Input: part model. Units: mm. Frame: model coordinates. Face numbers are marked on the shaded views. A direction names the side the tool comes from. Give positions to 0.01 mm unless a question says otherwise; leave off trailing zeros. Write each loop counter-clockwise with the first axis right and the second up, starting at its lowest first coordinate (ties: lowest second). Pieces come first, ordered by that corner, then holes. Notation, with made-up numbers: (53.5, 58) - (108.5, 58) arc R20 ccw to (108.5, 85) - close; hole circle Ø3 at (79, -39). An arc over 180 degrees is marked (long way). Use a Markdown table: item, result. Add a question column.
1. Material intervals for probe 1 along Y at (x, z) = (0, -8.75); probe 2 along X at (y, z) = (-0.75, -11.25); probe 3 along Y at (x, z) = (1, -0.5), sorted ascending.
2. Pin query (flat end, axial travel): pin 1 (1.2 mm diameter, centred on x = 0, z = -1, fed in from -Y); pin 2 (3 mm diameter, centred on x = 0, z = -7, fed in from +Y); pin 3 (0.9 mm diameter, centred on x = 0, z = -1, fed in from +Y). Return the tip coordinate at first contact, or that it passes through.
3. Section query B-B, the plane z = -7. Return loops of the section in (x, y), plus the area to 3 significant figures.
4. Mould query, pull axis Y, two halves, no side actions, for the marked faces 3, 4 and 5. Classes: released by +Y, released by -Y, zero draft, split by the parting line, or undercut.
5. Set-up query: the marked faces 1 and 2. Return all of +Z, -Z, +X, -X, +Y, -Y with unobstructed straight access to the full face (end or side cutting, diameter ignored); none if empty.
```python
from build123d import *

# Parameters (mm, degrees)
SKETCH001_R     = 2.15
POCKET_DEPTH    = 3.119566
CHAMFER_SIZE    = 0.25
CHAMFER001_SIZE = 0.2


with BuildPart() as pocket:
    # Sketch003 → Revolution001 (revolve)
    with BuildSketch(Plane.XZ):
        Polygon((0, -2.118566), (1.15, -1.7), (1.15, 1), (0, 1), align=None)
    revolve(axis=Axis((0, 0, 0), (0, 0, 1)))

    # Sketch001 → Pocket (cut, through all)
    with BuildSketch(Plane(origin=(0, 0, 1), x_dir=(-1, 0, 0), z_dir=(0, 0, 1))):
        Circle(SKETCH001_R)
        Polygon((-0.57735, 1), (0.57735, 1), (1.154701, 0), (0.57735, -1), (-0.57735, -1), (-1.154701, 0), align=None, mode=Mode.SUBTRACT)
    extrude(amount=-POCKET_DEPTH, mode=Mode.SUBTRACT)


with BuildPart() as chamfer001:
    # Sketch → Revolution (revolve)
    with BuildSketch(Plane.XZ):
        Polygon((1.15, 0), (3.199999, 0), (1.5, -1.7), (1.5, -12), (0, -12), (0, -1.150001), align=None)
    revolve(axis=Axis((0, 0, 0), (0, 0, 1)))

    # Cut: cut Pocket
    add(pocket.part, mode=Mode.SUBTRACT)

    # Chamfer
    chamfer_edges = [chamfer001.edges().sort_by_distance(p)[0] for p in [
        (-3.199999, 0, 0),
    ]]
    chamfer(chamfer_edges, length=CHAMFER_SIZE)

    # Chamfer001
    chamfer001_edges = [chamfer001.edges().sort_by_distance(p)[0] for p in [
        (-1.5, 0, -12),
    ]]
    chamfer(chamfer001_edges, length=CHAMFER001_SIZE)


solid = chamfer001.part
```
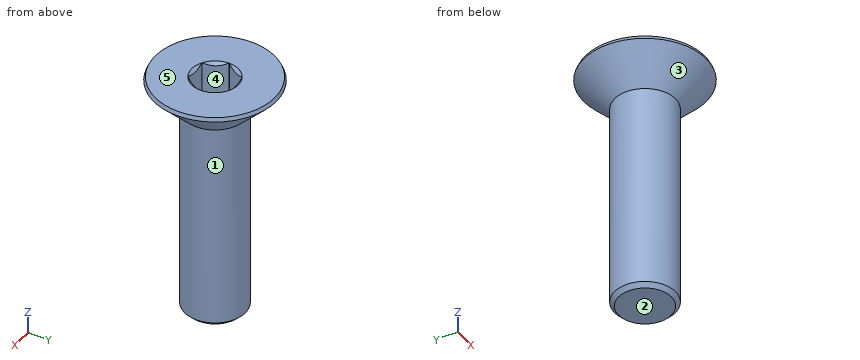
Result sheet:
| question | item | result |
|---|---|---|
| 1 | probe 1 | y = -1.5 to 1.5 |
| 1 | probe 2 | x = -1.3 to 1.3 |
| 1 | probe 3 | y = -2.51 to -0.27, 0.27 to 2.51 |
| 2 | pin 1 | stops at y = -2.8 |
| 2 | pin 2 | stops at y = 1.5 |
| 2 | pin 3 | stops at y = 2.65 |
| 3 | outline | circle Ø3 at (0, 0) |
| 3 | area | 7.07 mm² |
| 4 | face 3 | split by the parting line |
| 4 | face 4 | undercut |
| 4 | face 5 | zero draft |
| 5 | face 1 | -Z |
| 5 | face 2 | -Z, +X, -X, +Y, -Y |
